```python
from build123d import *

# Parameters (mm, degrees)
BOSS_EXTRUDE10_DEPTH = 3.5
BOSS_EXTRUDE15_DEPTH = 1.25
SKETCH1_17_W         = 34.75
SKETCH1_17_H         = 2.924143722
BOSS_EXTRUDE17_DEPTH = 29.25
BOSS_EXTRUDE18_DEPTH = 1.25
SKETCH2_9_R          = 1.75
BOSS_EXTRUDE19_DEPTH = 1.75
BOSS_EXTRUDE19_TAPER = 4
FILLET1_R            = 2


with BuildPart() as part:
    # Sketch1 → Boss-Extrude10 (new body)
    with BuildSketch(Plane.XY):
        with BuildLine():
            ThreePointArc((0, 6.75), (-3.375, 3.375), (0, 0))
            Line((0, 0), (14.75, 0))
            Line((14.75, 0), (14.75, 6.75))
            Line((14.75, 6.75), (0, 6.75))
        make_face()
        with BuildLine():
            ThreePointArc((0, 0.5), (-2.875, 3.375), (0, 6.25))
            Line((0, 6.25), (12.265078429, 5.016721387))
            ThreePointArc((12.265078429, 5.016721387), (13.75, 3.375), (12.265078429, 1.733278613))
            Line((12.265078429, 1.733278613), (0, 0.5))
        make_face(mode=Mode.SUBTRACT)
    extrude(amount=BOSS_EXTRUDE10_DEPTH)

    # Sketch1<16> → Boss-Extrude15 (add)
    with BuildSketch(Plane.XY):
        with BuildLine():
            Line((0, 6.25), (-0.57238697, 6.192445325))
            ThreePointArc((-0.57238697, 6.192445325), (-2.875, 3.375), (-0.57238697, 0.557554675))
            Line((-0.57238697, 0.557554675), (0, 0.5))
            Line((0, 0.5), (12.265078429, 1.733278613))
            ThreePointArc((12.265078429, 1.733278613), (13.75, 3.375), (12.265078429, 5.016721387))
            Line((12.265078429, 5.016721387), (0, 6.25))
        make_face()
    extrude(amount=BOSS_EXTRUDE15_DEPTH)

    # Sketch1<17> → Boss-Extrude17 (add)
    with BuildSketch(Plane.XY):
        with Locations((32.125, 3.375)):
            Rectangle(SKETCH1_17_W, SKETCH1_17_H)
    extrude(amount=BOSS_EXTRUDE17_DEPTH)

    # Sketch2 → Boss-Extrude18 (add)
    with BuildSketch(Plane.XY.offset(29.25)):
        Polygon((13.5, 5.875), (-8.061356684, 5.875), (-8.061356684, 0.875), (14.75, 0.875), (14.75, 5.875), align=None)
    extrude(amount=-BOSS_EXTRUDE18_DEPTH)

    # Sketch2<9> → Boss-Extrude19 (add)
    with BuildSketch(Plane.XY.offset(29.25)):
        with Locations((0, 3.375)):
            Circle(SKETCH2_9_R)
    extrude(amount=BOSS_EXTRUDE19_DEPTH, taper=BOSS_EXTRUDE19_TAPER)

    # Fillet1
    # the kernel refuses this fillet: 2 mm, written as the material it adds along each edge
    with BuildSketch(Plane(origin=(14.75, 1.912928139, 0), x_dir=(0, -1, 0), z_dir=(0, 0, 1))) as fillet1_piece_1:
        with BuildLine():
            CenterArc((2, 1.998103724), FILLET1_R, 180, 87.504786267)
            Line((0, 1.998103724), (0, 0))
            Line((0, 0), (1.912928139, 0))
        make_face()
    extrude(amount=3.5)
    with BuildSketch(Plane(origin=(14.75, 4.837071861, 0), x_dir=(1, 0, 0), z_dir=(0, 0, 1))) as fillet1_piece_2:
        with BuildLine():
            CenterArc((1.998103724, 2), FILLET1_R, 182.495213733, 87.504786267)
            Line((0, 1.912928139), (0, 0))
            Line((0, 0), (1.998103724, 0))
        make_face()
    extrude(amount=3.5)
    with BuildSketch(Plane(origin=(14.75, 1.912928139, 28), x_dir=(1, 0, 0), z_dir=(0, 0, 1))) as fillet1_piece_3:
        with BuildLine():
            CenterArc((1.753401761, -2), FILLET1_R, 90, 61.246917848)
            Line((0, -1.037928139), (0, 0))
            Line((0, 0), (1.753401761, 0))
        make_face()
    extrude(amount=1.25)
    with BuildSketch(Plane(origin=(14.75, 4.837071861, 28), x_dir=(1, 0, 0), z_dir=(0, 0, 1))) as fillet1_piece_4:
        with BuildLine():
            CenterArc((1.753401761, 2), FILLET1_R, 208.753082152, 61.246917848)
            Line((0, 1.037928139), (0, 0))
            Line((0, 0), (1.753401761, 0))
        make_face()
    extrude(amount=1.25)


solid = part.part
```
The listing builds one solid part. Answer for the finished solid, in the listing's coordinates (mm). A direction names the side the tool comes from. Round coordinates to 2 decimals unless told otherwise and drop trailing zeros. Loops run counter-clockwise (first coordinate to the right, second up) from the corner with the lowest first, then second, coordinate; pieces in that order, holes last. Notation, with made-up numbers: (57.5, 1) - (93.5, 1) arc R15 cw to (93.5, 28) - close; hole circle Ø2 at (41, 11). An arc over 180 degrees is marked (long way). Return JSON: item names as keys, results as strings. Group by question number.
1. The part is cut by section A-A on x = 2.5. Determine the outline of the cut face in (y, z) (3 decimals), then the cut area to 3 significant figures.
2. The mould has two halves that part along X. Classify faces 5 (the cylindrical face through (-2.874, 3.312, 2.114)), 6 (the conical face through (0.9, 4.787, 30.332)), 7 (the cylindrical face through (13.75, 3.41, 2.36)), 8 (the flat face through (14.75, 3, 16)): pulls with the +X half, pulls with the -X half, needs draft (parallel to the pull), parting line crosses it, or undercut.
3. Each of these flat-tipped pins is pushed along its axis until it touches: P1, Ø1.5, axis at y = 5.5, z = 9.5, coming from the +X side; P2, Ø1.4, axis at x = -0.5, z = 28.5, coming from the +Y side (3 decimals); P3, Ø14.5, axis at x = 27.5, z = 20.5, coming from the +Y side; P4, Ø3, axis at y = 3.5, z = 19.5, coming from the -X side. Where does it stop, or does it pass through?
4. Consider probe 1 along Z at (x, y) = (11, 1); probe 2 along Z at (x, y) = (-1.5, 5.75); probe 3 along X at (y, z) = (2.5, 12.5). Determine where each line is inside the solid, lowest interval first.
5. The part is cut by section C-C on x = 18. Determine the outline of the cut face in (y, z).
6. Which of the six approach directions +Z, -Z, +X, -X, +Y, -Y give full straight-line access (tool end or side, diameter ignored) to faces 1 (the cylindrical face through (15.498, 1.642, 28.616)), 2 (the flat face through (4, 5.875, 29)), 3 (the cylindrical face through (-3.374, 3.449, 1.726)), 4 (the flat face through (6.05, 5.64, 2.36))?
7. The part is cut by section B-B on z = 21.5. Determine the outline of the cut face in (x, y), then the cut area to 3 significant figures.
Resolved:
{
 "1": {"outline": "(0, 0) - (6.75, 0) - (6.75, 3.5) - (5.999, 3.5) - (5.999, 1.25) - (0.751, 1.25) - (0.751, 3.5) - (0, 3.5) - close; (0.875, 28) - (5.875, 28) - (5.875, 29.25) - (0.875, 29.25) - close", "area": "18.1 mm²"},
 "2": {"face 5": "undercut", "face 6": "parting line crosses it", "face 7": "undercut", "face 8": "pulls with the -X half"},
 "3": {"P1": "stops at x = 49.5", "P2": "stops at y = 5.875", "P3": "stops at y = 4.84", "P4": "stops at x = 14.75"},
 "4": {"probe 1": "z = 0 to 3.5, 28 to 29.25", "probe 2": "z = 0 to 1.25, 28 to 29.25", "probe 3": "x = 14.75 to 49.5"},
 "5": {"outline": "(1.91, 0) - (4.84, 0) - (4.84, 29.25) - (1.91, 29.25) - close"},
 "6": {"face 1": "+Z, +X, -Y", "face 2": "+Z, +X, -X, +Y", "face 3": "-Z, -X", "face 4": "none"},
 "7": {"outline": "(14.75, 1.91) - (49.5, 1.91) - (49.5, 4.84) - (14.75, 4.84) - close", "area": "102 mm²"}
}
